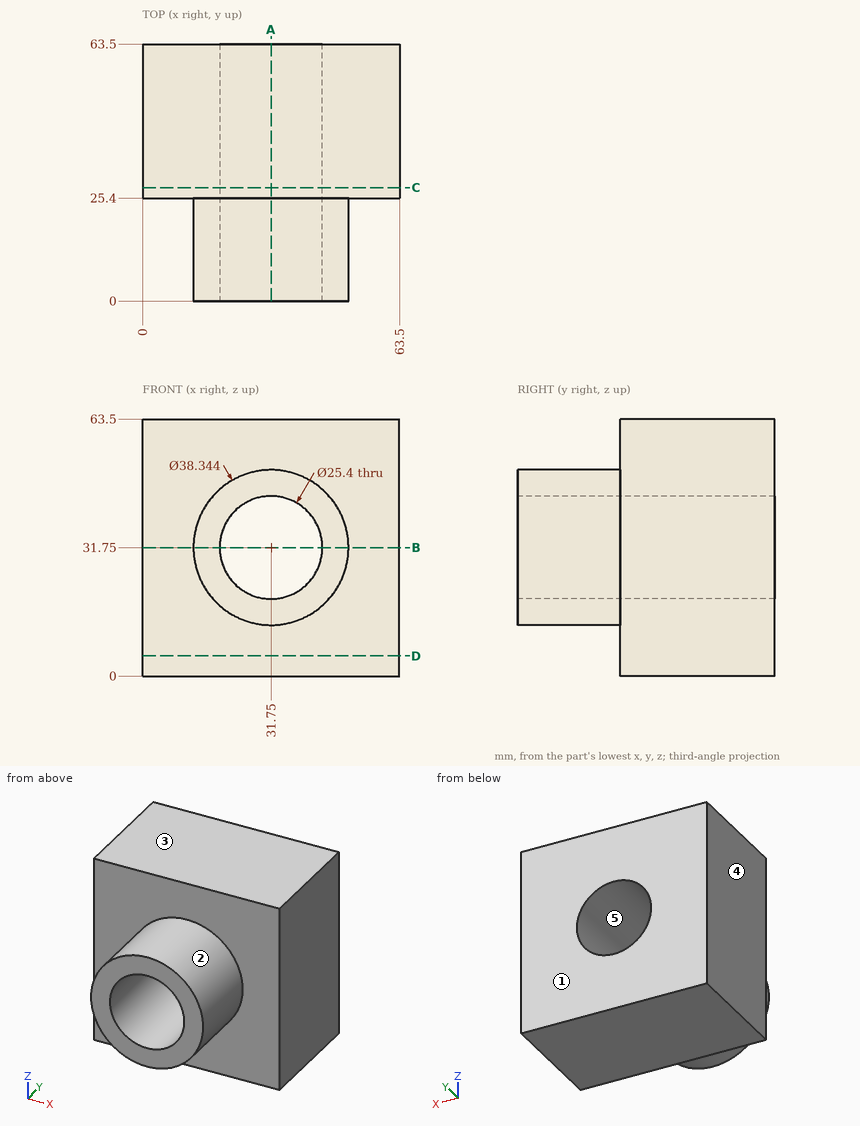
Geometry check sheet. Reference: drawing and pictorial views, mm from the part's lowest x, y, z. A direction names the side the tool comes from. Round coordinates to 2 decimals unless told otherwise and drop trailing zeros. Loops run counter-clockwise (first coordinate to the right, second up) from the corner with the lowest first, then second, coordinate; pieces in that order, holes last.
1. Sectioned sample at A-A on x = 31.75. Record the boundary of the cut face in (y, z).
2. Sectioned sample at C-C on y = 28. Record the boundary of the cut face in (x, z).
3. Gauge pin test, flat ends, axial feed: pin 1 Ø5 at (x, y) = (45, 17.5) entering from -Z (1 decimal); pin 2 Ø1 at (x, z) = (50.5, 21.5) entering from -Y; pin 3 Ø2 at (x, z) = (22, 30.5) entering from -Y; pin 4 Ø6 at (y, z) = (15, 37.5) entering from +X. Record the tip position at first contact, or that the pin passes through.
4. Sectioned sample at B-B on z = 31.75. Record the boundary of the cut face in (x, y).
5. Scan lines: probe 1 along X at (y, z) = (29, 31); probe 2 along Y at (x, z) = (56.5, 41). Record each from-to range of solid material in increasing order.
6. Sectioned sample at D-D on z = 5. Record the boundary of the cut face in (x, y), and give its area (3 significant figures).
7. Set-up check for the marked faces 1 and 2: record each of +Z, -Z, +X, -X, +Y, -Y from which the full face is reachable in a straight line by a thin tool's end or side.
8. Mould release check, pull along X, two halves, no side actions. Record for the marked faces 3, 4 and 5: released by +X, released by -X, zero draft, split by the parting line, or undercut.
Recorded:
1. outline: (0, 12.58) - (25.4, 12.58) - (25.4, 0) - (63.5, 0) - (63.5, 19.05) - (0, 19.05) - close; (0, 44.45) - (63.5, 44.45) - (63.5, 63.5) - (25.4, 63.5) - (25.4, 50.92) - (0, 50.92) - close
2. outline: (0, 0) - (63.5, 0) - (63.5, 63.5) - (0, 63.5) - close; hole circle Ø25.4 at (31.75, 31.75)
3. pin 1: stops at z = 15.9
3. pin 2: stops at y = 25.4
3. pin 3: passes through
3. pin 4: stops at x = 50.72
4. outline: (0, 25.4) - (12.58, 25.4) - (12.58, 0) - (19.05, 0) - (19.05, 63.5) - (0, 63.5) - close; (44.45, 0) - (50.92, 0) - (50.92, 25.4) - (63.5, 25.4) - (63.5, 63.5) - (44.45, 63.5) - close
5. probe 1: x = 0 to 19.07, 44.43 to 63.5
5. probe 2: y = 25.4 to 63.5
6. outline: (0, 25.4) - (63.5, 25.4) - (63.5, 63.5) - (0, 63.5) - close
6. area: 2,420 mm2
7. face 1: +Z, -Z, +X, -X, +Y
7. face 2: -Y
8. face 3: zero draft
8. face 4: released by -X
8. face 5: undercut
